Geometry: final body of the model. Coordinates: model frame, mm. A direction names the side the tool comes from. Coordinates: 2 decimals unless noted, no trailing zeros. Write each loop counter-clockwise with the first axis right and the second up, starting at its lowest first coordinate (ties: lowest second). Pieces come first, ordered by that corner, then holes. Notation, with made-up numbers: (-16, -0.5) -> (20, -0.5) arc R24 cw to (20, 16.5) -> close; hole circle Ø4 at (-18, 53). An arc over 180 degrees is marked (long way). One line per item, written item: value.
Autodesk Inventor part; units mm, degrees
ref_plane "YZ Plane" through (0, 0, 0) normal (1, 0, 0) x (0, 1, 0)
ref_plane "XZ Plane" through (0, 0, 0) normal (0, 1, 0) x (-1, 0, 0)
ref_plane "XY Plane" through (0, 0, 0) normal (0, 0, 1) x (1, 0, 0)
sketch "スケッチ1" plane through (0, 0, 0) normal (0, 0, 1) x (1, 0, 0)
  line L0 (-6.5, 3.5) -> (6.5, 3.5)
  line L1 (6.5, 3.5) -> (6.5, -3.5)
  line L2 (6.5, -3.5) -> (-6.5, -3.5)
  line L3 (-6.5, -3.5) -> (-6.5, 3.5)
  line L4 (-6.5, 3.5) -> (6.5, -3.5) construction
  line L5 (6.5, 3.5) -> (-6.5, -3.5) construction
  line L6 (5.5, 3.5) -> (5.5, -3.5)
  line L7 (0.5, 3.5) -> (0.5, -3.5)
  line L8 (-0.5, 3.5) -> (-0.5, -3.5)
  line L9 (-5.5, 3.5) -> (-5.5, -3.5)
  line L10 (0, -4.9) -> (0, 4.9)
  circle A0 centre (-3, 0) radius 2.5
  circle A1 centre (3, 0) radius 2.5
  line L11 (-6.5, -2.5) -> (6.5, -2.5)
  line L12 (-6.5, 2.5) -> (6.5, 2.5)
  line L13 (-9.1, 0) -> (9.1, 0)
  line L14 (-5.5, 2.5) -> (-0.5, -2.5) construction
  line L15 (-5.5, -2.5) -> (-0.5, 2.5) construction
  line L16 (5.5, 2.5) -> (0.5, -2.5) construction
  line L17 (5.5, -2.5) -> (0.5, 2.5) construction
  point P0 (0, 0)
  point P1 (0, 0)
  point P2 (3, 0)
  point P3 (-3, 0)
  point P4 (0, -3.5)
  point P5 (0, 3.5)
  dimension "d2" = 1
  dimension "d3" = 1
  dimension "d4" = 1
  dimension "d5" = 5
  dimension "d8" = 5
  dimension "d9" = 5
  dimension "d10" = 1
  dimension "d11" = 5
extrude "押し出し1" add sketch "スケッチ1" against normal blind 6.5
extrude "押し出し2" add sketch "スケッチ1" along normal blind 3 contours L0 L9 L12 L3 | L0 L8 L12 L9 | L12 L9 L13 L3 | L0 L10 L12 L8 | L12 A0 L9 | L13 L9 L11 L3 | L12 L10 L13 L8 | L8 A0 L12 | A0 L11 L9 | L13 A0 | A0 L13 | L11 L9 L2 L3 | L13 L10 L11 L8 | L8 L11 A0 | L11 L8 L2 L9 | L11 L10 L2 L8
extrude "押し出し3" cut sketch "スケッチ1" along normal mid plane 20 contours L13 A0 | A0 L13 | L13 A1 | A1 L13
chamfer "面取り1" distance 1 angle 45 4 edges at (-6.5, 3.5, -1.75) (6.5, 3.5, -3.25) (6.5, -3.5, -3.25) (-6.5, -3.5, -1.75)
ref_plane "作業平面1" through (-5.5, -3.5, -6.5) normal (0, -1, 0) x (1, 0, 0)
sketch "スケッチ2" plane through (-5.5, -3.5, -6.5) normal (0, -1, 0) x (1, 0, 0)
  line L0 (0, 0) -> (0, 9.5)
  line L1 (11, 0) -> (0, 0)
  line L2 (11, 6.5) -> (11, 0)
  line L3 (5.5, 6.5) -> (11, 6.5)
  line L4 (5.5, 6.5) -> (5.5, 9.5)
  line L5 (0, 9.5) -> (5.5, 9.5)
  line L6 (0.5, 5.75) -> (10.5, 5.75)
  line L7 (10.5, 5.75) -> (10.5, 0.75)
  line L8 (10.5, 0.75) -> (0.5, 0.75)
  line L9 (0.5, 0.75) -> (0.5, 5.75)
  line L10 (0, 0) -> (0, 9.5)
  line L11 (11, 0) -> (12, 0)
  line L12 (0, 6.5) -> (11, 0) construction
  line L13 (5, 0) -> (0, 0)
  line L14 (12, 6.5) -> (11, 6.5)
  line L15 (0, 0) -> (11, 6.5) construction
  line L16 (12, 6.5) -> (-1, 6.5)
  line L17 (0.5, 5.75) -> (10.5, 0.75) construction
  line L18 (0.5, 0.75) -> (10.5, 5.75) construction
  point P0 (6.5, 6.5)
  point P1 (5.5, 3.25)
  dimension "d25" = 5
  dimension "d26" = 10
extrude "押し出し4" add sketch "スケッチ2" along normal blind 0.1 contours L6 L7 L8 L9
ref_plane "作業平面2" through (-6.5, -2.5, 3) normal (-1, 0, 0) x (0, 0, 1)
properties part number "sensorholder_3"
(1) Section C-C (z = 2). Return the cut outline in (x, y).
Responses:
outline: (-6.5, -2.5) -> (-5.5, -3.5) -> (0, -3.5) -> (0, 3.5) -> (-5.5, 3.5) -> (-6.5, 2.5) -> close; hole circle Ø5 at (-3, 0)
(2) Line query: line 1 (X direction, y = 2.25, z = -2); line 2 (X direction, y = -1, z = -3); line 3 (Y direction, x = -3, z = -3.25). Output: solid intervals per line, ascending. Write a range as [from, to].
Responses:
line 1: x = [-6.5, -4.09], [-1.91, 1.91], [4.09, 6.5]
line 2: x = [-6.5, -5.29], [-0.71, 0.71], [5.29, 6.5]
line 3: y = [-3.6, -2.5], [2.5, 3.5]
(3) Section D-D (z = -4). Return the cut outline in (x, y).
Responses:
outline: (-6.5, -2.5) -> (-5.5, -3.5) -> (-5, -3.5) -> (-5, -3.6) -> (5, -3.6) -> (5, -3.5) -> (5.5, -3.5) -> (6.5, -2.5) -> (6.5, 2.5) -> (5.5, 3.5) -> (-5.5, 3.5) -> (-6.5, 2.5) -> close; hole circle Ø5 at (-3, 0); hole circle Ø5 at (3, 0)
(4) Pull-direction query (X, two-part tool) for faces 3 (the flat face through (0, 3.5, -3)), 4 (the cylindrical face through (1, -1.5, -3.2)), 5 (the flat face through (-6.5, 0, -2)), 6 (the flat face through (6, -3, -3)); classes: released by +X, released by -X, zero draft, split by the parting line, or undercut.
Responses:
face 3: zero draft
face 4: undercut
face 5: released by -X
face 6: released by +X
(5) Reachability of faces 1 (the flat face through (-6, -3, -2)), 2 (the flat face through (1, 2, 0)) from +Z, -Z, +X, -X, +Y, -Y: full face, straight path, thin tool, end or side. Return the list, or none.
Responses:
face 1: +Z, -Z, -X, -Y
face 2: +Z, +X, +Y, -Y
(6) Section B-B (x = 4.5). Return the cut outline in (y, z), then the cut area to 3 significant figures.
Responses:
outline: (-3.6, -5.75) -> (-3.5, -5.75) -> (-3.5, -6.5) -> (-2, -6.5) -> (-2, 0) -> (-3.5, 0) -> (-3.5, -0.75) -> (-3.6, -0.75) -> close; (2, -6.5) -> (3.5, -6.5) -> (3.5, 0) -> (2, 0) -> close
area: 20.0 mm2
(7) First-contact query: pin 1 (1.5 mm diameter, centred on x = 4.5, z = -0.5, fed in from -Y); pin 2 (0.9 mm diameter, centred on y = -0.5, z = 2, fed in from +X). Flat tips, straight axial feed; report the tip coordinate or a pass-through.
Responses:
pin 1: stops at y = -3.6
pin 2: stops at x = 0
(8) Section A-A (y = 2). Return the cut outline in (x, z), then the cut area to 3 significant figures.
Responses:
outline: (-6.5, -6.5) -> (-4.5, -6.5) -> (-4.5, 3) -> (-6.5, 3) -> close; (-1.5, -6.5) -> (1.5, -6.5) -> (1.5, 0) -> (0, 0) -> (0, 3) -> (-1.5, 3) -> close; (4.5, -6.5) -> (6.5, -6.5) -> (6.5, 0) -> (4.5, 0) -> close
area: 56.0 mm2
